Read the model definition and answer for the solid it produces. Units are mm, in the model's axes. Coordinates: 2 decimals unless noted, no trailing zeros. Loops run counter-clockwise (first coordinate to the right, second up) from the corner with the lowest first, then second, coordinate; pieces in that order, holes last. Notation, with made-up numbers: (85, 38.5) -> (125, 38.5) arc R24 ccw to (125, 53.5) -> close; hole circle Ø6 at (85, -31). An arc over 180 degrees is marked (long way). Answer as CSV lines item,"result".
Autodesk Inventor part; units mm, degrees
ref_plane "YZ Plane" through (0, 0, 0) normal (1, 0, 0) x (0, 1, 0)
ref_plane "XZ Plane" through (0, 0, 0) normal (0, 1, 0) x (-1, 0, 0)
ref_plane "XY Plane" through (0, 0, 0) normal (0, 0, 1) x (1, 0, 0)
sketch "Sketch1" plane through (0, 0, 0) normal (1, 0, 0) x (0, 1, 0)
  line L0 (0, 0) -> (0, -300)
  line L1 (0, -300) -> (0, 0)
  line L2 (0, 0) -> (0, 300)
  line L3 (0, 300) -> (150, 300)
  line L4 (150, 300) -> (150, 200)
  line L5 (150, 200) -> (0, 200)
  line L6 (0, 200) -> (0, 300)
  line L7 (0, -300) -> (150, -300)
  line L8 (150, -300) -> (150, -200)
  line L9 (150, -200) -> (0, -200)
  line L10 (0, -200) -> (0, -300)
  dimension "d0" = 300
  dimension "d1" = 300
  dimension "d2" = 150
  dimension "d3" = 100
  dimension "d4" = 150
  dimension "d5" = 100
extrude "Extrusion1" add sketch "Sketch1" along normal blind 20
sketch "Sketch2" plane through (0, 0, -200) normal (0, 0, 1) x (1, 0, 0)
  point P0 (0, 0)
sketch "Sketch6" plane through (0, 0, -200) normal (0, 0, 1) x (1, 0, 0)
  line L0 (0, 150) -> (20, 150)
  line L1 (10, 150) -> (10, 0)
  line L2 (10, 0) -> (10, 150)
  line L3 (10, 75) -> (10, 150)
  line L4 (10, 112.5) -> (10, 75)
  line L5 (10, 0) -> (10, 75)
  circle A0 centre (10, 112.5) radius 7.5
  circle A1 centre (10, 75) radius 7.5
  circle A2 centre (10, 37.5) radius 7.5
  point P0 (0, 0)
  dimension "d13" = 15
  dimension "d14" = 15
  dimension "d15" = 15
extrude "Extrusion3" add sketch "Sketch6" along normal blind 400.125
properties part number "2"
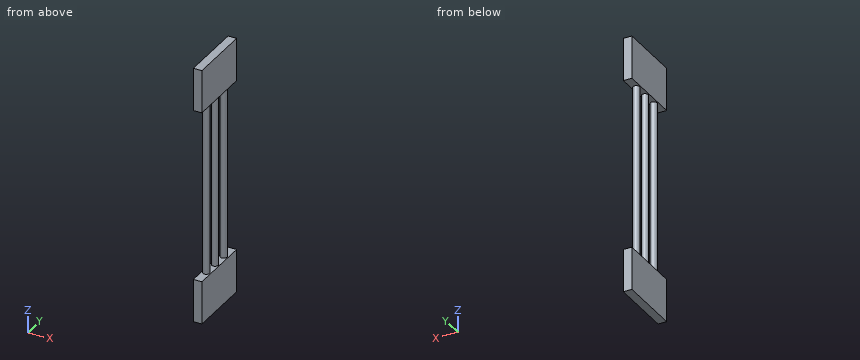
Q1. A cutting plane is placed at C-C, the plane z = -94. Write down the section's boundary in (x, y), and give its area (3 significant figures).
Results:
outline,"circle Ø15 at (10, 37.5); circle Ø15 at (10, 75); circle Ø15 at (10, 112.5)"
area,"530 mm²"
Q2. A cutting plane is placed at A-A, the plane x = 5.5. Write down the section's boundary in (y, z).
Results:
outline,"(0, -300) -> (150, -300) -> (150, -200) -> (118.5, -200) -> (118.5, 200) -> (150, 200) -> (150, 300) -> (0, 300) -> (0, 200) -> (31.5, 200) -> (31.5, -200) -> (0, -200) -> close; hole (43.5, -200) -> (69, -200) -> (69, 200) -> (43.5, 200) -> close; hole (81, -200) -> (106.5, -200) -> (106.5, 200) -> (81, 200) -> close"
Q3. A cutting plane is placed at B-B, the plane y = 128.5. Write down the section's boundary in (x, z).
Results:
outline,"(0, -300) -> (20, -300) -> (20, -200) -> (0, -200) -> close; (0, 200) -> (20, 200) -> (20, 300) -> (0, 300) -> close"
Q4. Given pin 1 Ø1.5 at (x, z) = (14, 107.5) entering from -Y; pin 2 Ø6 at (y, z) = (45, 24) entering from +X; pin 3 Ø5 at (x, z) = (11.5, -8) entering from +Y, each flat-ended and moving along its own axis, determine where each tip first touches the part or whether it passes through.
Results:
pin 1,"stops at y = 30.74"
pin 2,"stops at x = 16"
pin 3,"stops at y = 120"
Q5. Find the intervals of material crossed by probe 1 along Z at (x, y) = (5, 47.5); probe 2 along Y at (x, z) = (7, 166.5); probe 3 along Y at (x, z) = (16, -159.5), in increasing order. Write a range as [from, to].
Results:
probe 1,"z = [-300, -200], [200, 300]"
probe 2,"y = [30.63, 44.37], [68.13, 81.87], [105.63, 119.37]"
probe 3,"y = [33, 42], [70.5, 79.5], [108, 117]"
